Design review of the part shown in the three views and the two pictorial views. Dimensions are in mm from the part's minimum x, y and z. A direction names the side the tool comes from. Round coordinates to 2 decimals unless told otherwise and drop trailing zeros. Write each loop counter-clockwise with the first axis right and the second up, starting at its lowest first coordinate (ties: lowest second). Pieces come first, ordered by that corner, then holes. Notation, with made-up numbers: (-20, -8) - (38, -8) arc R27 cw to (38, 18) - close; hole circle Ø7 at (63.5, -19.75). An arc over 180 degrees is marked (long way). Use one line per item in the form item = value.
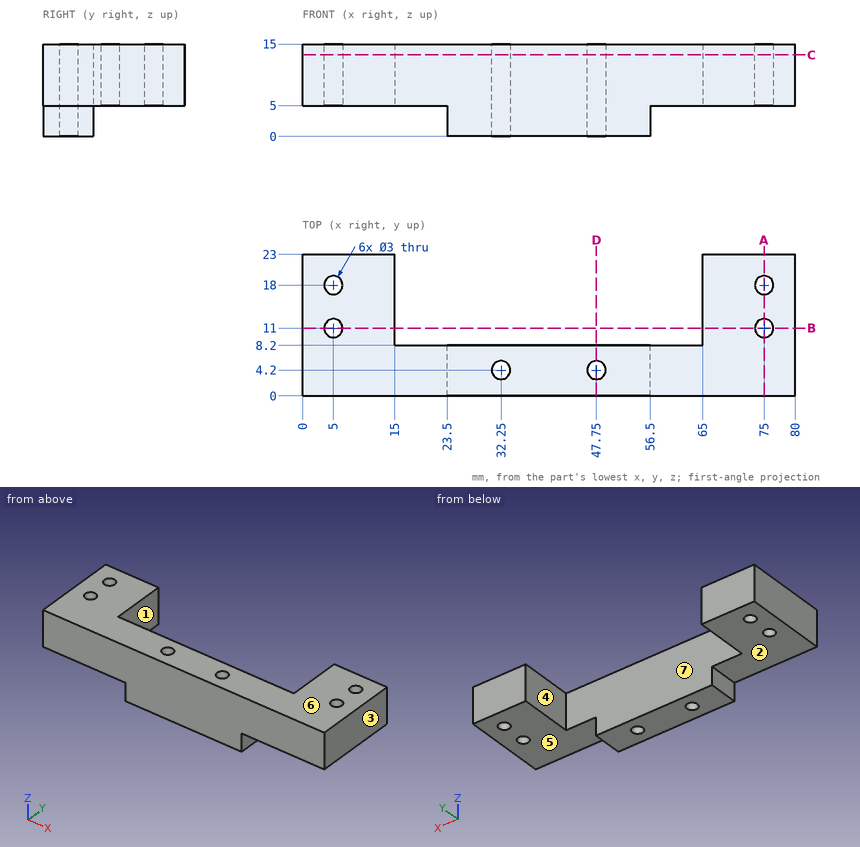
Q1. We need section B-B on y = 11. Write out the cut boundary in (x, z), then the cut area to 3 significant figures.
Calculated:
outline = (0, 5) - (3.5, 5) - (3.5, 15) - (0, 15) - close; (6.5, 5) - (15, 5) - (15, 15) - (6.5, 15) - close; (65, 5) - (73.5, 5) - (73.5, 15) - (65, 15) - close; (76.5, 5) - (80, 5) - (80, 15) - (76.5, 15) - close
area = 240 mm2
Q2. Machinability: for the marked faces 5, 6 and 7, which of the approach directions +Z, -Z, +X, -X, +Y, -Y give a long, thin tool a straight path to every point of the face, cutting with its end or side? Answer none if there is none.
Calculated:
face_5 = -Z, +X, +Y, -Y
face_6 = +Z, +X, -X, +Y, -Y
face_7 = +Z, -Z, +Y
Q3. For P1, Ø1.5, axis at x = 27.5, z = 8, coming from the +Y side; P2, Ø7, axis at x = 74, y = 16.5, coming from the -Z side; P3, Ø1.5, axis at y = 6, z = 3.5, coming from the -X side, all flat-tipped, find the tip position at first contact; note any pin that passes through.
Calculated:
P1 = 8.2
P2 = 5
P3 = 23.5
Q4. We need section D-D on x = 47.75. Write out the cut boundary in (y, z), then the cut area to 3 significant figures.
Calculated:
outline = (0, 0) - (2.7, 0) - (2.7, 15) - (0, 15) - close; (5.7, 0) - (8.2, 0) - (8.2, 15) - (5.7, 15) - close
area = 78.0 mm2
Q5. To check wall thickness, follow line 1 along Y through (x, z) = (5, 12.5); line 2 along X through (y, z) = (8.5, 7.5); line 3 along X through (y, z) = (4.5, 5.5). State the ranges of each line that lie inside material, in increasing order. Write a range as from..to.
Calculated:
line_1 = 0..9.5, 12.5..16.5, 19.5..23
line_2 = 0..15, 65..80
line_3 = 0..30.78, 33.72..46.28, 49.22..80
Q6. We need section A-A on x = 75. Write out the cut boundary in (y, z).
Calculated:
outline = (0, 5) - (9.5, 5) - (9.5, 15) - (0, 15) - close; (12.5, 5) - (16.5, 5) - (16.5, 15) - (12.5, 15) - close; (19.5, 5) - (23, 5) - (23, 15) - (19.5, 15) - close
Q7. Draft analysis for pull direction X (two halves, no side actions). For the marked faces 1, 2, 3 and 4, state which applies: released by +X, released by -X, zero draft, split by the parting line, or undercut.
Calculated:
face_1 = undercut
face_2 = zero draft
face_3 = released by +X
face_4 = undercut
Q8. We need section C-C on z = 13.25. Write out the cut boundary in (x, y).
Calculated:
outline = (0, 0) - (80, 0) - (80, 23) - (65, 23) - (65, 8.2) - (15, 8.2) - (15, 23) - (0, 23) - close; hole circle Ø3 at (5, 11); hole circle Ø3 at (5, 18); hole circle Ø3 at (32.25, 4.2); hole circle Ø3 at (47.75, 4.2); hole circle Ø3 at (75, 11); hole circle Ø3 at (75, 18)
